from build123d import *

# Parameters (mm, degrees)
CUT_EXTRUDE1_DEPTH = 1
SCALE1_SCALE       = 1.7


with BuildPart() as part:
    # Sketch1 → Revolve1 (revolve)
    with BuildSketch(Plane.XY):
        with BuildLine():
            Line((0, 0), (0, 1.43))
            ThreePointArc((0, 1.43), (1.238500708, 2.474899998), (2.814888985, 2.85))
            Line((2.814888985, 2.85), (3.164888985, 2.85))
            Line((3.164888985, 2.85), (3.164888985, 1.5))
            Line((3.164888985, 1.5), (40.164888985, 1.5))
            Line((40.164888985, 1.5), (40.164888985, 0))
            Line((40.164888985, 0), (0, 0))
        make_face()
    revolve(axis=Axis((0, 0, 0), (1, 0, 0)))

    # Sketch2 → Cut-Extrude1 (cut)
    with BuildSketch(Plane.ZY):
        Polygon((1, 0), (0.5, 0.866025404), (-0.5, 0.866025404), (-1, 0), (-0.5, -0.866025404), (0.5, -0.866025404), align=None)
    extrude(amount=-CUT_EXTRUDE1_DEPTH, mode=Mode.SUBTRACT)


with BuildPart() as part_1:
    # Scale1: scaled about (17.990832775, 0, 0)
    add(part.part.scale(SCALE1_SCALE).moved(Location((-12.593582942, 0, 0))))


solid = part_1.part
Here's how the part is built. I have some questions about the finished solid (model axes, mm). A direction names the side the tool comes from. Coordinates: 2 decimals unless noted, no trailing zeros. Order: outer loops, then holes, each group sorted by start corner. A loop starts at its lowest first (then second) coordinate and runs counter-clockwise, first axis right, second up. Notation, with made-up numbers: (68, 51) -> (75, 51) arc R6 cw to (75, 56) -> close; hole circle Ø3 at (-38, 68). An arc over 180 degrees is marked (long way). Answer in a Markdown table with one row per item.
(1) I want a section at A-A on x = 38. List the corners of the cut face in (y, z) for me, then the cut area to 3 significant figures.
Answer key:
| item | result |
|---|---|
| outline | circle Ø5.1 at (0, 0) |
| area | 20.4 mm^2 |
(2) Please list where these lines run through material, in increasing order: probe 1 along Y at (x, z) = (1, -0.75); probe 2 along Y at (x, z) = (23, -0.25); probe 3 along X at (y, z) = (0.25, 0.75).
Answer key:
| item | result |
|---|---|
| probe 1 | -2.44 to 2.44 |
| probe 2 | -2.54 to 2.54 |
| probe 3 | -10.89 to 55.69 |
(3) Will these pins go through, and if not, where does the flat tip stop? pin 1 Ø1.5 at (x, y) = (22.5, -2) entering from +Z; pin 2 Ø1.9 at (x, z) = (-11.5, 0.5) entering from -Y; pin 3 Ø0.8 at (x, z) = (-11.5, 0) entering from +Y.
Answer key:
| item | result |
|---|---|
| pin 1 | z = 2.22 |
| pin 2 | y = -4.15 |
| pin 3 | y = 3.85 |
(4) On a 3-axis mill with a long thin cutter (end or side, diameter ignored), from which of +Z, -Z, +X, -X, +Y, -Y can I reach the whole of each face in a straight line? I mean faces 1 (the face through (55.687, 0, 0)), 2 (the face through (24.68, 1.18, -2.26)), 3 (the face through (-11.755, -0.746, 1.269)). Say none if no direction works.
Answer key:
| item | result |
|---|---|
| face 1 | +Z, -Z, +X, +Y, -Y |
| face 2 | +X |
| face 3 | -X |
(5) Thinking about a two-plate mould opening in X: for faces 4 (the face through (-12.594, -2, 0)), 5 (the face through (-11.76, 0.73, 1.28)), 6 (the face through (-7.213, 2, -2)), which applies, +X half, -X half, draft (parallel to the pull), parting line (faces both ways), or undercut?
Answer key:
| item | result |
|---|---|
| face 4 | -X half |
| face 5 | draft |
| face 6 | +X half |
